CAD build for the part. Positions are in the model's coordinates, mm. A direction names the side the tool comes from. Give positions to 0.01 mm unless a question says otherwise; leave off trailing zeros. Order: outer loops, then holes, each group sorted by start corner. A loop starts at its lowest first (then second) coordinate and runs counter-clockwise, first axis right, second up.
```python
from build123d import *

# Parameters (mm, degrees)
BOSS_EXTRUDE1_DEPTH = 1.3
SKETCH2_W           = 20
SKETCH2_H           = 1.4
SKETCH2_W_2         = 1.4
SKETCH2_H_2         = 10
BOSS_EXTRUDE2_DEPTH = 1.3
SKETCH3_W           = 6
SKETCH3_H           = 1.4
SKETCH3_W_2         = 1.4
SKETCH3_H_2         = 6
CUT_EXTRUDE1_DEPTH  = 46.678384543
SKETCH4_R           = 3.1
CUT_EXTRUDE2_DEPTH  = 46.678384543


with BuildPart() as part:
    # Sketch1 → Boss-Extrude1 (new body)
    with BuildSketch(Plane(origin=(0, 0, 0), x_dir=(0, 0, -1), z_dir=(1, 0, 0))):
        with BuildLine():
            Line((-31.228581667, 0), (-31.228581667, 20))
            Line((-31.228581667, 20), (-17.420583246, 22.310666482))
            Line((-17.420583246, 22.310666482), (-17.420583246, 19.310666482))
            Line((-17.420583246, 19.310666482), (-3.612584824, 19.310666482))
            Line((-3.612584824, 19.310666482), (-3.612584824, 33.310666482))
            Line((-3.612584824, 33.310666482), (4.898619689, 33.310666482))
            ThreePointArc((4.898619689, 33.310666482), (12.292551865, 30.690758286), (16.387415176, 24))
            Line((16.387415176, 24), (16.387415176, 0))
            Line((16.387415176, 0), (0, 0))
            Line((0, 0), (-31.228581667, 0))
        make_face()
    extrude(amount=BOSS_EXTRUDE1_DEPTH)

    # Sketch2 → Boss-Extrude2 (add)
    with BuildSketch(Plane(origin=(1.3, 0, 0), x_dir=(0, 0, -1), z_dir=(1, 0, 0))):
        with Locations((-15.612584824, -0.7)):
            Rectangle(SKETCH2_W, SKETCH2_H)
        with Locations((17.087415176, 10)):
            Rectangle(SKETCH2_W_2, SKETCH2_H_2)
    extrude(amount=-BOSS_EXTRUDE2_DEPTH)

    # Sketch3 → Cut-Extrude1 (cut, through all)
    with BuildSketch(Plane(origin=(1.3, 0, 0), x_dir=(0, 0, -1), z_dir=(1, 0, 0))):
        with Locations((1.387415176, 30.610666482)):
            Rectangle(SKETCH3_W, SKETCH3_H)
        with Locations((11.687415176, 22)):
            Rectangle(SKETCH3_W_2, SKETCH3_H_2)
    extrude(amount=-CUT_EXTRUDE1_DEPTH, mode=Mode.SUBTRACT)

    # Sketch4 → Cut-Extrude2 (cut, through all)
    with BuildSketch(Plane(origin=(1.3, 0, 0), x_dir=(0, 0, -1), z_dir=(1, 0, 0))):
        with Locations((-12.612584824, 4.5)):
            Circle(SKETCH4_R)
    extrude(amount=-CUT_EXTRUDE2_DEPTH, mode=Mode.SUBTRACT)


solid = part.part
```
Item 1: Drop flat-ended pins along their axis: pin 1 Ø0.6 at (x, y) = (1, 21) entering from -Z; pin 2 Ø5 at (y, z) = (4, 21.5) entering from -X; pin 3 Ø0.6 at (x, y) = (1, 30.5) entering from +Z; pin 4 Ø0.6 at (x, z) = (1, -17) entering from -Y. Give the stop position or say it passes through.
Item 2: Two-plate mould, pull along Y, no slides. Class faces 4 (the face through (0.641, 30.761, -12.205)), 5 (the face through (1, 3, -16.387)), 6 (the face through (1, 25, -12)): released by +Y, released by -Y, zero draft, split by the parting line, or undercut.
Item 3: Slice it at A-A (y = 4.5). Give the cut face in (x, z), and give its area (3 significant figures).
Item 4: Tool access for faces 1 (the face through (1, 21, 17.421)), 2 (the face through (1, -1, 5.613)), 3 (the face through (1, 29.911, -1)): list every direction of +Z, -Z, +X, -X, +Y, -Y with a clear straight run to the whole face (end or side of a thin tool).
Item 5: Slice it at D-D (z = -6). Give the cut face in (x, y).
Item 6: Wall check: L1, parallel to Y at x = 0.5, z = -2.5; L2, parallel to Z at x = 0.35, y = 23; L3, parallel to Y at x = 0.7, z = 12. Give the ranges that are in metal, low to high.
Item 7: Slice it at B-B (x = 0.5). Give the cut face in (y, z), and give its area (3 significant figures).
Item 8: Slice it at C-C (y = 17.5). Give the cut face in (x, z).
A:
1. pin 1: stops at z = -16.39
1. pin 2: stops at x = 0
1. pin 3: stops at z = 3.61
1. pin 4: stops at y = 5
2. face 4: released by +Y
2. face 5: zero draft
2. face 6: undercut
3. outline: (0, -16.39) - (1.3, -16.39) - (1.3, 9.51) - (0, 9.51) - close; (0, 15.71) - (1.3, 15.71) - (1.3, 31.23) - (0, 31.23) - close
3. area: 53.8 mm2
4. face 1: +X, -X, +Y
4. face 2: -Z, +X, -X, -Y
4. face 3: +X, -X
5. outline: (0, 0) - (1.3, 0) - (1.3, 33.26) - (0, 33.26) - close
6. L1: y = 0 to 29.91, 31.31 to 33.31
6. L2: z = -16.39 to -12.39, -10.99 to 3.61
6. L3: y = -1.4 to 1.46, 7.54 to 19.31
7. outline: (-1.4, 5.61) - (0, 5.61) - (0, -16.39) - (5, -16.39) - (5, -17.79) - (15, -17.79) - (15, -16.39) - (24, -16.39) arc R11.74 ccw to (33.31, -4.9) - (33.31, 3.61) - (19.31, 3.61) - (19.31, 17.42) - (22.31, 17.42) - (20, 31.23) - (0, 31.23) - (0, 25.61) - (-1.4, 25.61) - close; hole circle Ø6.2 at (4.5, 12.61); hole (19, -12.39) - (25, -12.39) - (25, -10.99) - (19, -10.99) - close; hole (29.91, -4.39) - (31.31, -4.39) - (31.31, 1.61) - (29.91, 1.61) - close
7. area: 1,190 mm2
8. outline: (0, -16.39) - (1.3, -16.39) - (1.3, 31.23) - (0, 31.23) - close
